Part model, mm, in its own coordinate system. Give positions to 0.01 mm unless a question says otherwise; leave off trailing zeros. Write each loop counter-clockwise with the first axis right and the second up, starting at its lowest first coordinate (ties: lowest second). Pieces come first, ordered by that corner, then holes. Notation, with made-up numbers: M 44,10 L 48,10 A29 cw 48,36 Z; hole C 89.5,-11.75 d11. An arc over 180 degrees is marked long. Use a Markdown table: item, result.
```python
from build123d import *

# Parameters (mm, degrees)
SKETCH1_W          = 4
SKETCH1_H          = 4
CHAMFER1_SIZE      = 0.4
CHAMFER1_SIZE2     = 0.230940108
SKETCH2_R          = 2.5
CUT_EXTRUDE1_DEPTH = 2


with BuildPart() as part:
    # Sketch1 → Revolve1 (revolve)
    with BuildSketch(Plane(origin=(0, 0, 0), x_dir=(1, 0, 0), z_dir=(0, 1, 0))):
        with Locations((2, 0)):
            Rectangle(SKETCH1_W, SKETCH1_H)
    revolve(axis=Axis((0, 0, -141.429107981), (0, 0, 1)))

    # Chamfer1
    chamfer1_edges = [part.edges().sort_by_distance(p)[0] for p in [
        (-4, 0, -2),
    ]]
    chamfer1_side = [part.faces().sort_by_distance(p)[0] for p in [
        (-4, 0, 0),
    ]]
    chamfer(chamfer1_edges, length=CHAMFER1_SIZE, length2=CHAMFER1_SIZE2, reference=chamfer1_side[0])

    # Sketch2 → Cut-Extrude1 (cut)
    with BuildSketch(Plane.XY.offset(2)):
        Circle(SKETCH2_R)
    extrude(amount=-CUT_EXTRUDE1_DEPTH, mode=Mode.SUBTRACT)


solid = part.part
```
1. Drill centre lines: L1, parallel to Y at x = 0, z = 1; L2, parallel to X at y = -2.25, z = 1.85. Where is each one in solid material? Low to high.
Findings below:
| item | result |
|---|---|
| L1 | -4 to -2.5, 2.5 to 4 |
| L2 | -3.31 to -1.09, 1.09 to 3.31 |
2. Two-plate mould, pull along X, no slides. Class faces 1 (the cylindrical face through (-0.54, -2.44, 1.01)), 2 (the cylindrical face through (-0.867, -3.905, 0.175)), 3 (the flat face through (0, 0, 0)), 4 (the flat face through (-2, 2, 2)): released by +X, released by -X, zero draft, split by the parting line, or undercut.
Findings below:
| item | result |
|---|---|
| face 1 | undercut |
| face 2 | split by the parting line |
| face 3 | undercut |
| face 4 | zero draft |
3. Drop flat-ended pins along their axis: P1, Ø1, axis at y = -1, z = 1, coming from the -X side; P2, Ø1.5, axis at y = 2, z = 0, coming from the -X side. Give the stop position or say it passes through.
Findings below:
| item | result |
|---|---|
| P1 | x = -3.97 |
| P2 | x = -3.8 |
4. Cut at A-A, the plane x = 0. Give the cut face in (y, z), then the cut area to 3 significant figures.
Findings below:
| item | result |
|---|---|
| outline | M -4,-1.6 L -3.77,-2 L 3.77,-2 L 4,-1.6 L 4,2 L 2.5,2 L 2.5,0 L -2.5,0 L -2.5,2 L -4,2 Z |
| area | 21.9 mm2 |
5. Cut at C-C, the plane z = 1.05. Give the cut face in (x, y).
Findings below:
| item | result |
|---|---|
| outline | C 0,0 d8; hole C 0,0 d5 |
